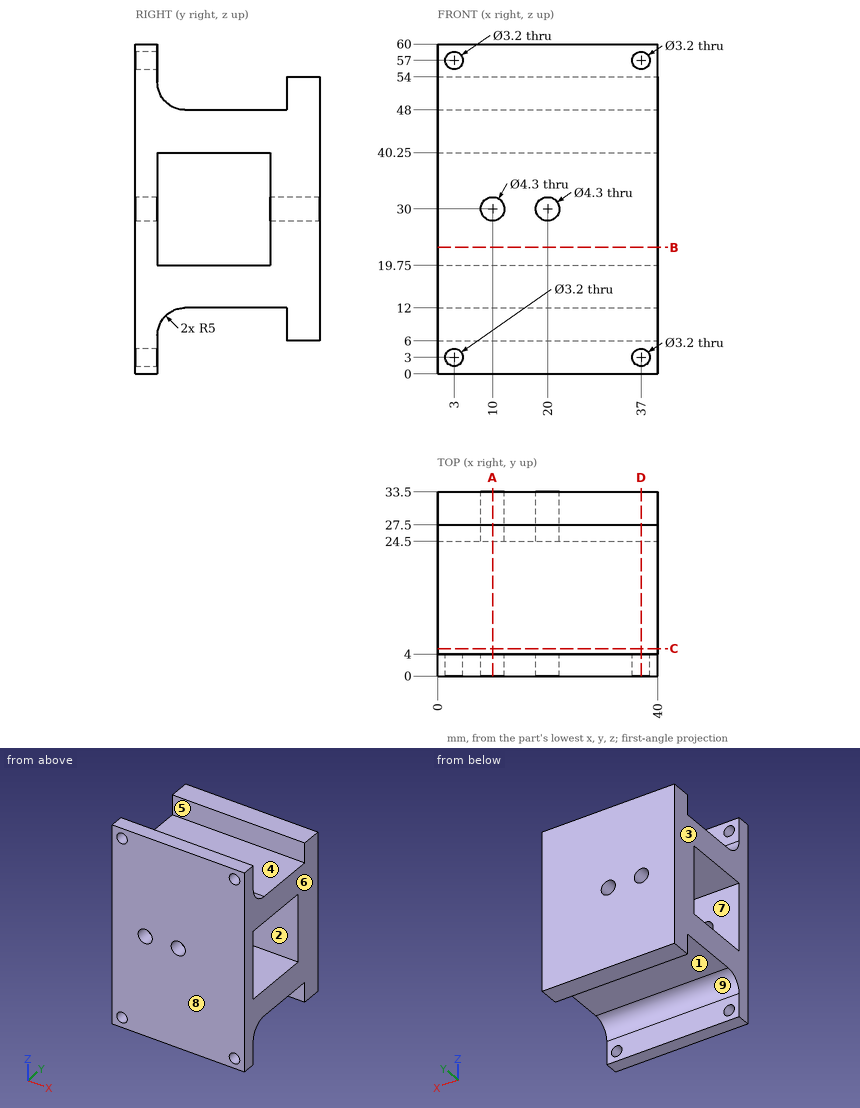
Check sheet for the drawn part. Datum: minimum x, y, z corner. Units: mm. A direction names the side the tool comes from. Coordinates: 2 decimals unless noted, no trailing zeros. Loops run counter-clockwise (first coordinate to the right, second up) from the corner with the lowest first, then second, coordinate; pieces in that order, holes last. Notation, with made-up numbers: (-14, -7.75) -> (21, -7.75) arc R11 cw to (21, -0.75) -> close; hole circle Ø5 at (39.25, 47). An arc over 180 degrees is marked (long way). Write each question's results on one line, items separated by ' | '.
Item 1: Section check A-A, the plane x = 10. Enter the section's corners in (y, z), plus the area to 3 significant figures.
Found:
outline: (0, 0) -> (4, 0) -> (4, 7) arc R5 cw to (9, 12) -> (27.5, 12) -> (27.5, 6) -> (33.5, 6) -> (33.5, 27.85) -> (24.5, 27.85) -> (24.5, 19.75) -> (4, 19.75) -> (4, 27.85) -> (0, 27.85) -> close; (0, 32.15) -> (4, 32.15) -> (4, 40.25) -> (24.5, 40.25) -> (24.5, 32.15) -> (33.5, 32.15) -> (33.5, 54) -> (27.5, 54) -> (27.5, 48) -> (9, 48) arc R5 cw to (4, 53) -> (4, 60) -> (0, 60) -> close | area: 909 mm2
Item 2: Section check B-B, the plane z = 23. Enter the section's corners in (x, y).
Found:
outline: (0, 0) -> (40, 0) -> (40, 4) -> (0, 4) -> close; (0, 24.5) -> (40, 24.5) -> (40, 33.5) -> (0, 33.5) -> close
Item 3: Tool access check on the marked faces 5, 6, 7, 8 and 9. Record the directions out of +Z, -Z, +X, -X, +Y, -Y that give a thin tool (end or side, any length) a straight path to the whole face; none if there is none.
Found:
face 5: +Z, +X, -X | face 6: +Z, -Z, +X, +Y, -Y | face 7: +X, -X | face 8: +Z, -Z, +X, -X, -Y | face 9: -Z, +X, -X
Item 4: Material ranges on L1, parallel to X at y = 1, z = 3; L2, parallel to X at y = 1, z = 30; L3, parallel to Z at x = 25, y = 16, recorded low to high.
Found:
L1: x = 0 to 1.4, 4.6 to 35.4, 38.6 to 40 | L2: x = 0 to 7.85, 12.15 to 17.85, 22.15 to 40 | L3: z = 12 to 19.75, 40.25 to 48
Item 5: Section check C-C, the plane y = 5. Enter the section's corners in (x, z).
Found:
outline: (0, 10) -> (40, 10) -> (40, 19.75) -> (0, 19.75) -> close; (0, 40.25) -> (40, 40.25) -> (40, 50) -> (0, 50) -> close
Item 6: Section check D-D, the plane x = 37. Enter the section's corners in (y, z), plus the area to 3 significant figures.
Found:
outline: (0, 0) -> (4, 0) -> (4, 1.4) -> (0, 1.4) -> close; (0, 4.6) -> (4, 4.6) -> (4, 7) arc R5 cw to (9, 12) -> (27.5, 12) -> (27.5, 6) -> (33.5, 6) -> (33.5, 54) -> (27.5, 54) -> (27.5, 48) -> (9, 48) arc R5 cw to (4, 53) -> (4, 55.4) -> (0, 55.4) -> close; (0, 58.6) -> (4, 58.6) -> (4, 60) -> (0, 60) -> close; hole (4, 19.75) -> (24.5, 19.75) -> (24.5, 40.25) -> (4, 40.25) -> close | area: 939 mm2
Item 7: Gauge pin test, flat ends, axial feed: pin 1 (4 mm diameter, centred on x = 3, z = 3, fed in from +Y); pin 2 (12 mm diameter, centred on x = 10.5, y = 17.5, fed in from -Z); pin 3 (5 mm diameter, centred on x = 25, y = 30, fed in from +Z). Record the tip position at first contact, or that the pin passes through.
Found:
pin 1: stops at y = 4 | pin 2: stops at z = 12 | pin 3: stops at z = 54
Item 8: Mould release check, pull along Z, two halves, no side actions. Record for the marked faces 1, 2, 3 and 4: +Z half, -Z half, draft (parallel to the pull), parting line (faces both ways), or undercut.
Found:
face 1: -Z half | face 2: undercut | face 3: draft | face 4: +Z half
